Verification items for the finished model (mm, model axes). A direction names the side the tool comes from. Give positions to 0.01 mm unless a question says otherwise; leave off trailing zeros. Write each loop counter-clockwise with the first axis right and the second up, starting at its lowest first coordinate (ties: lowest second). Pieces come first, ordered by that corner, then holes. Notation, with made-up numbers: (-24.75, 12) -> (9.25, 12) arc R12 cw to (9.25, 25) -> close; hole circle Ø2 at (-29.5, 63). An arc over 180 degrees is marked (long way). Answer as CSV lines item,"result".
```python
from build123d import *

# Parameters (mm, degrees)
SKETCH1_R                = 15.175
SKETCH1_R_2              = 6.5
BOSS_EXTRUDE1_DEPTH      = 3
SKETCH2_R                = 10.5
SKETCH2_R_2              = 9.75
BOSS_EXTRUDE2_DEPTH      = 3
M2_CLEARANCE_HOLE1_D     = 2.2
M2_CLEARANCE_HOLE1_DEPTH = 10
M2_CLEARANCE_HOLE1_TIP   = 0.660946681


with BuildPart() as part:
    # Sketch1 → Boss-Extrude1 (new body)
    with BuildSketch(Plane.XY):
        Circle(SKETCH1_R)
        Circle(SKETCH1_R_2, mode=Mode.SUBTRACT)
    extrude(amount=BOSS_EXTRUDE1_DEPTH)

    # Sketch2 → Boss-Extrude2 (add)
    with BuildSketch(Plane.XY.offset(3)):
        Circle(SKETCH2_R)
        Circle(SKETCH2_R_2, mode=Mode.SUBTRACT)
    extrude(amount=BOSS_EXTRUDE2_DEPTH)

    # M2 Clearance Hole1
    with Locations(Plane(origin=(0, 0, 0), x_dir=(-1, 0, 0), z_dir=(0, 0, -1))):
        with Locations((0, 12.8375), (12.8375, 0), (0, -12.8375), (-12.8375, 0)):
            Hole(M2_CLEARANCE_HOLE1_D / 2, depth=M2_CLEARANCE_HOLE1_DEPTH)
            with Locations((0, 0, -(M2_CLEARANCE_HOLE1_DEPTH + M2_CLEARANCE_HOLE1_TIP / 2))):  # 118° drill point
                Cone(0, M2_CLEARANCE_HOLE1_D / 2, M2_CLEARANCE_HOLE1_TIP, mode=Mode.SUBTRACT)


solid = part.part
```
1) Tool access check on faces 1 (the flat face through (-4, -10, 3)), 2 (the cylindrical face through (14.474, 4.558, 1.479)). Record the directions out of +Z, -Z, +X, -X, +Y, -Y that give a thin tool (end or side, any length) a straight path to the whole face; none if there is none.
Reported:
face 1,"+Z"
face 2,"+Z, -Z"
2) Section check C-C (z = 3.6). Record the boundary of the cut face in (x, y).
Reported:
outline,"circle Ø21 at (0, 0); hole circle Ø19.5 at (0, 0)"
3) Depth check by flat-ended pin: pin 1 (1 mm diameter, centred on x = -8.5, z = 3, fed in from -Y) (3 decimals); pin 2 (2 mm diameter, centred on x = 0, y = 12.84, fed in from +Z); pin 3 (4 mm diameter, centred on x = 10, y = -10.5, fed in from +Z). Enter the tip coordinate at first touch or a pass-through.
Reported:
pin 1,"y = -12.895"
pin 2,"through"
pin 3,"z = 3"
4) Section check D-D (y = -3.5). Record the boundary of the cut face in (x, z), and give its area (3 significant figures).
Reported:
outline,"(-14.77, 0) -> (-5.48, 0) -> (-5.48, 3) -> (-9.1, 3) -> (-9.1, 6) -> (-9.9, 6) -> (-9.9, 3) -> (-14.77, 3) -> close; (5.48, 0) -> (14.77, 0) -> (14.77, 3) -> (9.9, 3) -> (9.9, 6) -> (9.1, 6) -> (9.1, 3) -> (5.48, 3) -> close"
area,"60.5 mm²"
5) Scan lines: line 1 along Y through (x, z) = (0, 1) (1 decimal); line 2 along Y through (x, z) = (0, 3.6); line 3 along Z through (x, y) = (11, -10). Record each from-to range of solid material in increasing order.
Reported:
line 1,"-15.2 to -13.9, -11.7 to -6.5, 6.5 to 11.7, 13.9 to 15.2"
line 2,"-10.5 to -9.75, 9.75 to 10.5"
line 3,"0 to 3"
6) Draft check along X on faces 3 (the flat face through (6, -8, 6)), 4 (the cylindrical face through (-12.25, 0.93, 1.52)), 5 (the cylindrical face through (10, 3.2, 4.5)). Enter one of: +X half, -X half, draft (parallel to the pull), parting line (faces both ways), or undercut.
Reported:
face 3,"draft"
face 4,"undercut"
face 5,"parting line"
7) Section check A-A (x = 0). State how many separate pieces and enclosed holes the cut face has, and give its area (4 significant figures).
Reported:
separate pieces,"4"
enclosed holes,"0"
area,"43.35 mm²"
